Here's how the part is built. I have some questions about the finished solid (model axes, mm). Face numbers are marked on the shaded views. A direction names the side the tool comes from. Round coordinates to 2 decimals unless told otherwise and drop trailing zeros. Order: outer loops, then holes, each group sorted by start corner. A loop starts at its lowest first (then second) coordinate and runs counter-clockwise, first axis right, second up. Notation, with made-up numbers: M -38,-34.75 L -30,-34.75 A21 ccw -30,-24.75 Z; hole C -19.5,73.5 d8. An arc over 180 degrees is marked long. Write item = value, one per line. Start each with the question number.
Item 1: I want a section at B-B, the plane y = -9. List the corners of the cut face in (x, z) for me, plus the area to 4 significant figures.
Item 2: For the marked faces 4 and 5, which set-ups out of +Z, -Z, +X, -X, +Y, -Y let a thin tool reach every point of the face, with its end or its side?
Item 3: I'm going to push flat-ended pins straight in: P1, Ø3.5, axis at y = 18, z = -7, coming from the -X side; P2, Ø1.6, axis at y = -4.5, z = -18, coming from the -X side; P3, Ø1.6, axis at x = -9, z = -12.5, coming from the +Y side; P4, Ø10, axis at x = -5, y = 10.5, coming from the -Z side. Where does each tip first touch, or does it pass through?
Item 4: I want a section at A-A, the plane x = 1.25. List the corners of the cut face in (y, z) for me (3 decimals), plus the area to 3 significant figures.
Item 5: I want a section at C-C, the plane x = -3. List the corners of the cut face in (y, z) for me (3 decimals), plus the area to 3 significant figures.
Item 6: I want a section at D-D, the plane y = 16. List the corners of the cut face in (x, z) for me, plus the area to 3 significant figures.
Item 7: We'd pull the mould along X, two halves only. Please class the marked faces 1, 2 and 3: pulls with the +X half, pulls with the -X half, needs draft (parallel to the pull), parting line crosses it, or undercut.
Item 8: Please list where these lines run through material, in increasing order: L1, parallel to X at y = -17, z = -17.5; L2, parallel to X at y = 1, z = -11.5; L3, parallel to Y at x = 1.5, z = -18.5 (3 decimals).
```python
from build123d import *

# Parameters (mm, degrees)
MAIN_EXTRUSION_DEPTH = 25


with BuildPart() as part:
    # Sk Main Extrusion → Main Extrusion (new body)
    with BuildSketch(Plane.XY):
        with BuildLine():
            Line((-3.83, 2.5328), (-11.31249103, 2.925083334))
            ThreePointArc((-11.31249103, 2.925083334), (-11.819967595, 3.366238681), (-11.514691833, 3.965369062))
            Line((-11.514691833, 3.965369062), (-10.100108722, 4.625))
            Line((-10.100108722, 4.625), (-9.58, 4.3))
            Line((-9.58, 4.3), (-8.08, 4.3))
            Line((-8.08, 4.3), (-5.474147193, 5))
            Line((-5.474147193, 5), (-4.934147193, 5))
            Line((-4.934147193, 5), (-4.23, 4.56))
            Line((-4.23, 4.56), (-4.23, 4.025))
            ThreePointArc((-4.23, 4.025), (-4.112842712, 3.742157288), (-3.83, 3.625))
            Line((-3.83, 3.625), (7.27, 3.625))
            Line((7.27, 3.625), (7.27, 5.120055168))
            Line((7.27, 5.120055168), (6.79886836, 5.120055168))
            ThreePointArc((6.79886836, 5.120055168), (5.9740485, 5.504367154), (5.638, 6.35))
            Line((5.638, 6.35), (5.638, 6.65))
            ThreePointArc((5.638, 6.65), (5.9740485, 7.495632846), (6.79886836, 7.879944832))
            Line((6.79886836, 7.879944832), (7.27, 7.879944832))
            Line((7.27, 7.879944832), (7.27, 15.470020156))
            Line((7.27, 15.470020156), (6.798058361, 15.470020156))
            ThreePointArc((6.798058361, 15.470020156), (5.938401057, 15.86929153), (5.588, 16.75))
            Line((5.588, 16.75), (5.588, 20))
            Line((5.588, 20), (7.52, 20))
            ThreePointArc((7.52, 20), (8.227106781, 19.707106781), (8.52, 19))
            Line((8.52, 19), (8.52, -19))
            ThreePointArc((8.52, -19), (8.227106781, -19.707106781), (7.52, -20))
            Line((7.52, -20), (5.588, -20))
            Line((5.588, -20), (5.588, -16.75))
            ThreePointArc((5.588, -16.75), (5.938401057, -15.86929153), (6.798058361, -15.470020156))
            Line((6.798058361, -15.470020156), (7.27, -15.470020156))
            Line((7.27, -15.470020156), (7.27, -7.879944832))
            Line((7.27, -7.879944832), (6.79886836, -7.879944832))
            ThreePointArc((6.79886836, -7.879944832), (5.9740485, -7.495632846), (5.638, -6.65))
            Line((5.638, -6.65), (5.638, -6.35))
            ThreePointArc((5.638, -6.35), (5.9740485, -5.504367154), (6.79886836, -5.120055168))
            Line((6.79886836, -5.120055168), (7.27, -5.120055168))
            Line((7.27, -5.120055168), (7.27, -3.625))
            Line((7.27, -3.625), (-3.83, -3.625))
            ThreePointArc((-3.83, -3.625), (-4.112842712, -3.742157288), (-4.23, -4.025))
            Line((-4.23, -4.025), (-4.23, -4.56))
            Line((-4.23, -4.56), (-4.934147193, -5))
            Line((-4.934147193, -5), (-5.474147193, -5))
            Line((-5.474147193, -5), (-8.08, -4.3))
            Line((-8.08, -4.3), (-9.58, -4.3))
            Line((-9.58, -4.3), (-10.100108722, -4.625))
            Line((-10.100108722, -4.625), (-11.514691833, -3.965369062))
            ThreePointArc((-11.514691833, -3.965369062), (-11.819967595, -3.366238681), (-11.31249103, -2.925083334))
            Line((-11.31249103, -2.925083334), (-3.83, -2.5328))
            Line((-3.83, -2.5328), (7.27, -2.339048779))
            Line((7.27, -2.339048779), (7.27, 2.339048779))
            Line((7.27, 2.339048779), (-3.83, 2.5328))
        make_face()
    extrude(amount=-MAIN_EXTRUSION_DEPTH)


solid = part.part
```
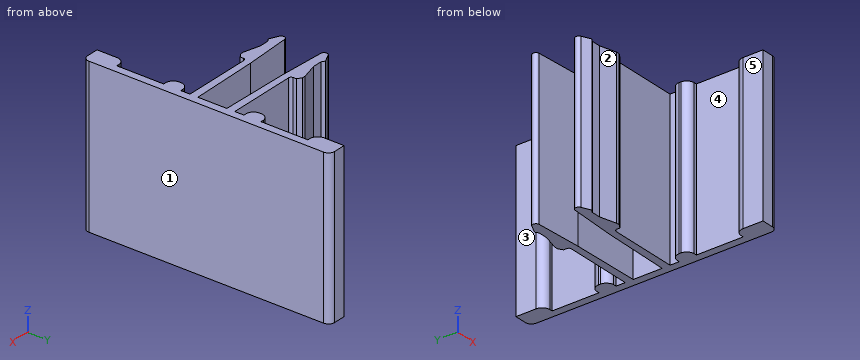
Filled in:
q1.outline = M 7.27,-25 L 8.52,-25 L 8.52,0 L 7.27,0 Z
q1.area = 31.25 mm^2
q2.face_4 = +Z, -Z, -X
q2.face_5 = +Z, -Z, -X, -Y
q3.P1 = 5.59
q3.P2 = -11.78
q3.P3 = 4.44
q3.P4 = through
q4.outline = M -3.625,-25 L -2.444,-25 L -2.444,0 L -3.625,0 Z; M 2.444,-25 L 3.625,-25 L 3.625,0 L 2.444,0 Z
q4.area = 59.0 mm^2
q5.outline = M -3.625,-25 L -2.518,-25 L -2.518,0 L -3.625,0 Z; M 2.518,-25 L 3.625,-25 L 3.625,0 L 2.518,0 Z
q5.area = 55.3 mm^2
q6.outline = M 5.83,-25 L 8.52,-25 L 8.52,0 L 5.83,0 Z
q6.area = 67.2 mm^2
q7.face_1 = pulls with the +X half
q7.face_2 = undercut
q7.face_3 = pulls with the -X half
q8.L1 = 5.59 to 8.52
q8.L2 = 7.27 to 8.52
q8.L3 = -3.625 to -2.44, 2.44 to 3.625
